from build123d import *

# Parameters (mm, degrees)
F0_W      = 60
F0_H      = 50
F1_DEPTH  = 20
F2_R      = 1
F3_DEPTH  = 1
F3_FACE_R = 1
F4_DEPTH  = 62


with BuildPart() as f1:
    # F0 (on Top) → F1 (new body)
    with BuildSketch(Plane.XY):
        with Locations((30, -25)):
            Rectangle(F0_W, F0_H)
    extrude(amount=F1_DEPTH)

    # F2 (on face) → F3 (join)
    with BuildSketch(Plane.YZ.offset(60)):
        with Locations((-5, 10)):
            Circle(F2_R)
    extrude(amount=F3_DEPTH)

    # F3_face (on face) → F4 (join)
    with BuildSketch(Plane(origin=(61, -5, 10), x_dir=(0, 1, 0), z_dir=(1, 0, 0))):
        Circle(F3_FACE_R)
    extrude(amount=-F4_DEPTH)


solid = f1.part
CAD build for the part. Positions are in the model's coordinates, mm. A direction names the side the tool comes from. Give positions to 0.01 mm unless a question says otherwise; leave off trailing zeros. Order: outer loops, then holes, each group sorted by start corner. A loop starts at its lowest first (then second) coordinate and runs counter-clockwise, first axis right, second up. Notation, with made-up numbers: (12.5, 60) -> (51.5, 60) arc R30 ccw to (51.5, 82) -> close; hole circle Ø6 at (54.5, -7). An arc over 180 degrees is marked (long way). Return JSON: item names as keys, results as strings.
Q1. Flat gauge pins, fed straight in: pin 1 (1.5 mm diameter, centred on y = -10, z = 9.5, fed in from +X); pin 2 (10 mm diameter, centred on y = -42, z = 11.5, fed in from -X). Where does each tip first touch, or does it go through?
Working result:
{"pin 1": "x = 60", "pin 2": "x = 0"}
Q2. Saw through at A-A (y = -5). Write the cut outline in (x, z), then the cut area to 3 significant figures.
Working result:
{"outline": "(-1, 9) -> (0, 9) -> (0, 0) -> (60, 0) -> (60, 9) -> (61, 9) -> (61, 11) -> (60, 11) -> (60, 20) -> (0, 20) -> (0, 11) -> (-1, 11) -> close", "area": "1,200 mm²"}
Q3. Saw through at B-B (z = 18.25). Write the cut outline in (x, y).
Working result:
{"outline": "(0, -50) -> (60, -50) -> (60, 0) -> (0, 0) -> close"}
Q4. Drill centre line: line 1 (X direction, y = -27, z = 10.75). Where is it in solid material? Low to high.
Working result:
{"line 1": "0 to 60"}
Q5. Which spindle directions (+Z, -Z, +X, -X, +Y, -Y) get a long thin tool onto all of the face, cutting with end or side? Do faces 1 (the face through (-0.49, -5.13, 10.99)), 2 (the face through (60.49, -5.13, 10.99)), 3 (the face through (30, -25, 20)). Say none if no direction does.
Working result:
{"face 1": "-X", "face 2": "+X", "face 3": "+Z, +X, -X, +Y, -Y"}
Q6. Saw through at C-C (y = -28). Write the cut outline in (x, z).
Working result:
{"outline": "(0, 0) -> (60, 0) -> (60, 20) -> (0, 20) -> close"}
